Part model, mm, in its own coordinate system. Round coordinates to 2 decimals unless told otherwise and drop trailing zeros. Order: outer loops, then holes, each group sorted by start corner. A loop starts at its lowest first (then second) coordinate and runs counter-clockwise, first axis right, second up. Notation, with made-up numbers: (-11, 47) - (47, 47) arc R22 ccw to (47, 54) - close; hole circle Ø8 at (88.25, 46). An arc over 180 degrees is marked (long way). Answer as a JSON object with one key per item and string values.
```python
from build123d import *

# Parameters (mm, degrees)
F0_R     = 7.75
F1_DEPTH = 4


with BuildPart() as f1:
    # F0 (on Front) → F1 (new body)
    with BuildSketch(Plane.XZ):
        with BuildLine():
            ThreePointArc((24.748737, -24.748737), (32.335784, -13.39392), (35, 0))
            ThreePointArc((35, 0), (32.335784, 13.39392), (24.748737, 24.748737))
            ThreePointArc((24.748737, 24.748737), (13.39392, 32.335784), (0, 35))
            ThreePointArc((0, 35), (-13.39392, 32.335784), (-24.748737, 24.748737))
            ThreePointArc((-24.748737, 24.748737), (-32.335784, 13.39392), (-35, 0))
            ThreePointArc((-35, 0), (-32.335784, -13.39392), (-24.748737, -24.748737))
            ThreePointArc((-24.748737, -24.748737), (-13.39392, -32.335784), (0, -35))
            ThreePointArc((0, -35), (13.39392, -32.335784), (24.748737, -24.748737))
        make_face()
        Circle(F0_R, mode=Mode.SUBTRACT)
        with BuildLine():
            ThreePointArc((-35, 0), (-32.335784, 13.39392), (-24.748737, 24.748737))
            Line((-24.748737, 24.748737), (-28.284271, 28.284271))
            ThreePointArc((-28.284271, 28.284271), (-31.954866, 24.060061), (-35, 19.364917))
            Line((-35, 19.364917), (-35, 0))
        make_face()
        with BuildLine():
            ThreePointArc((-24.748737, 24.748737), (-13.39392, 32.335784), (0, 35))
            Line((0, 35), (0, 40))
            ThreePointArc((0, 40), (-5.58247, 39.608535), (-11.055673, 38.441801))
            Line((-11.055673, 38.441801), (-24.748737, 24.748737))
        make_face()
        with BuildLine():
            Line((24.748737, 24.748737), (28.284271, 28.284271))
            ThreePointArc((28.284271, 28.284271), (24.060061, 31.954866), (19.364917, 35))
            Line((19.364917, 35), (0, 35))
            ThreePointArc((0, 35), (13.39392, 32.335784), (24.748737, 24.748737))
        make_face()
        with BuildLine():
            Line((35, 0), (40, 0))
            ThreePointArc((40, 0), (39.608535, 5.58247), (38.441801, 11.055673))
            Line((38.441801, 11.055673), (24.748737, 24.748737))
            ThreePointArc((24.748737, 24.748737), (32.335784, 13.39392), (35, 0))
        make_face()
        with BuildLine():
            ThreePointArc((28.284271, -28.284271), (31.954866, -24.060061), (35, -19.364917))
            Line((35, -19.364917), (35, 0))
            ThreePointArc((35, 0), (32.335784, -13.39392), (24.748737, -24.748737))
            Line((24.748737, -24.748737), (28.284271, -28.284271))
        make_face()
        with BuildLine():
            Line((11.055673, -38.441801), (24.748737, -24.748737))
            ThreePointArc((24.748737, -24.748737), (13.39392, -32.335784), (0, -35))
            Line((0, -35), (0, -40))
            ThreePointArc((0, -40), (5.58247, -39.608535), (11.055673, -38.441801))
        make_face()
        with BuildLine():
            Line((-19.364917, -35), (0, -35))
            ThreePointArc((0, -35), (-13.39392, -32.335784), (-24.748737, -24.748737))
            Line((-24.748737, -24.748737), (-28.284271, -28.284271))
            ThreePointArc((-28.284271, -28.284271), (-24.060061, -31.954866), (-19.364917, -35))
        make_face()
        with BuildLine():
            Line((-38.441801, -11.055673), (-24.748737, -24.748737))
            ThreePointArc((-24.748737, -24.748737), (-32.335784, -13.39392), (-35, 0))
            Line((-35, 0), (-40, 0))
            ThreePointArc((-40, 0), (-39.608535, -5.58247), (-38.441801, -11.055673))
        make_face()
    extrude(amount=F1_DEPTH)


solid = f1.part
```
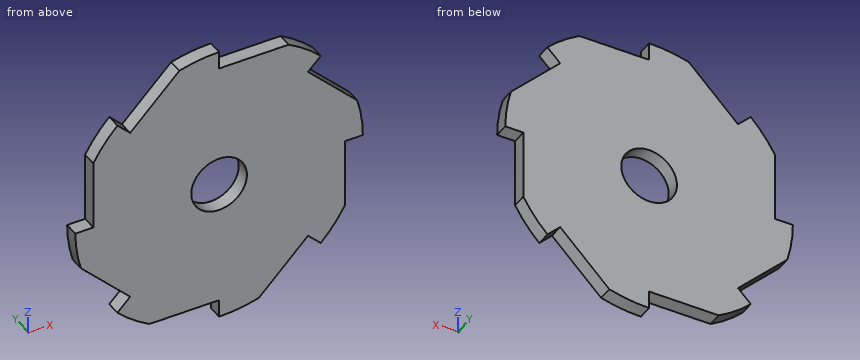
Item 1: Cut at A-A (y = -0.8). Write the cut outline in (x, z), plus the area to 3 significant figures.
Taken from the geometry:
{"outline": "(-40, 0) arc R40 ccw to (-38.44, -11.06) - (-24.75, -24.75) - (-28.28, -28.28) arc R40 ccw to (-19.36, -35) - (0, -35) - (0, -40) arc R40 ccw to (11.06, -38.44) - (24.75, -24.75) - (28.28, -28.28) arc R40 ccw to (35, -19.36) - (35, 0) - (40, 0) arc R40 ccw to (38.44, 11.06) - (24.75, 24.75) - (28.28, 28.28) arc R40 ccw to (19.36, 35) - (0, 35) - (0, 40) arc R40 ccw to (-11.06, 38.44) - (-24.75, 24.75) - (-28.28, 28.28) arc R40 ccw to (-35, 19.36) - (-35, 0) - close; hole circle Ø15.5 at (0, 0)", "area": "4,310 mm2"}
Item 2: Cut at B-B (x = 2). Write the cut outline in (y, z).
Taken from the geometry:
{"outline": "(-4, -39.95) - (0, -39.95) - (0, -7.49) - (-4, -7.49) - close; (-4, 7.49) - (0, 7.49) - (0, 35) - (-4, 35) - close"}
Item 3: Probe L1, parallel to X at y = -2.55, z = -28; L2, parallel to X at y = -3.05, z = 6; L3, parallel to Z at x = -2.5, y = -2.1. List the from-to ranges inside material, lowest first. Write a range as from..to.
Taken from the geometry:
{"L1": "-28..21.5, 28..28.57", "L2": "-35..-4.91, 4.91..39.55", "L3": "-35..-7.34, 7.34..39.92"}
Item 4: Cut at C-C (z = 1). Write the cut outline in (x, y), plus the area to 3 significant figures.
Taken from the geometry:
{"outline": "(-35, -4) - (-7.69, -4) - (-7.69, 0) - (-35, 0) - close; (7.69, -4) - (39.99, -4) - (39.99, 0) - (7.69, 0) - close", "area": "238 mm2"}
Item 5: Drop flat-ended pins along their axis: P1, Ø2, axis at x = -14, y = -1.5, coming from the -Z side; P2, Ø2, axis at x = 14, y = -1.5, coming from the +Z side; P3, Ø1, axis at y = -3.5, z = 8, coming from the -X side; P4, Ø9.5, axis at x = 0, z = 0, coming from the +Y side. Give the stop position or say it passes through.
Taken from the geometry:
{"P1": "z = -35", "P2": "z = 35", "P3": "x = -35", "P4": "through"}
Item 6: Cut at D-D (z = -9). Write the cut outline in (x, y).
Taken from the geometry:
{"outline": "(-38.97, -4) - (35, -4) - (35, 0) - (-38.97, 0) - close"}
